```python
from build123d import *

# Parameters (mm, degrees)
SKETCH1_W           = 101.6
SKETCH1_H           = 19.05
BOSS_EXTRUDE1_DEPTH = 3.175
SKETCH2_W           = 19.05
SKETCH2_H           = 19.05
BOSS_EXTRUDE2_DEPTH = 266.7
SKETCH4_W           = 114.3
SKETCH4_H           = 114.3
BOSS_EXTRUDE3_DEPTH = 76.2
SKETCH5_W           = 25.4
SKETCH5_H           = 38.1
CUT_EXTRUDE2_DEPTH  = 150.368
SKETCH7_OUTSIDE_W   = 192.692
SKETCH7_OUTSIDE_H   = 192.692
SKETCH7_OUTSIDE_W_2 = 101.6
SKETCH7_OUTSIDE_H_2 = 101.6
CUT_EXTRUDE3_DEPTH  = 50.8
SKETCH8_W           = 25.4
SKETCH8_H           = 33.866666666
CUT_EXTRUDE4_DEPTH  = 140.208
SKETCH9_W           = 114.3
SKETCH9_H           = 114.3
CUT_EXTRUDE5_DEPTH  = 12.7
FILLET2_R           = 6.35
SKETCH10_R          = 6.35
CUT_EXTRUDE6_DEPTH  = 12.7
SCALE1_SCALE        = 0.06
MOVE_FACE1_BY       = 0.380000002
MOVE_FACE1_2_BY     = 0.380000002
SKETCH12_R          = 0.5
BOSS_EXTRUDE4_DEPTH = 0.3
BOSS_EXTRUDE5_DEPTH = 0.3


with BuildPart() as part:
    # Sketch1 → Boss-Extrude1 (new body)
    with BuildSketch(Plane(origin=(0, 0, 0), x_dir=(0, 0, -1), z_dir=(1, 0, 0))):
        Rectangle(SKETCH1_W, SKETCH1_H)
    extrude(amount=BOSS_EXTRUDE1_DEPTH)

    # Sketch2 → Boss-Extrude2 (add)
    with BuildSketch(Plane(origin=(3.175, 0, 0), x_dir=(0, 0, -1), z_dir=(1, 0, 0))):
        Rectangle(SKETCH2_W, SKETCH2_H)
    extrude(amount=BOSS_EXTRUDE2_DEPTH)

    # Sketch4 → Boss-Extrude3 (add)
    with BuildSketch(Plane(origin=(269.875, 0, 0), x_dir=(0, 0, -1), z_dir=(1, 0, 0))):
        Rectangle(SKETCH4_W, SKETCH4_H)
    extrude(amount=BOSS_EXTRUDE3_DEPTH)

    # Sketch5 → Cut-Extrude2 (cut)
    with BuildSketch(Plane.XZ.offset(57.15)):
        with Locations((282.575, 38.1)):
            Rectangle(SKETCH5_W, SKETCH5_H)
        with Locations((282.575, -38.1)):
            Rectangle(SKETCH5_W, SKETCH5_H)
    extrude(amount=-CUT_EXTRUDE2_DEPTH, mode=Mode.SUBTRACT)

    # Sketch7 outside → Cut-Extrude3 (cut)
    with BuildSketch(Plane.ZY.offset(-269.875)):
        Rectangle(SKETCH7_OUTSIDE_W, SKETCH7_OUTSIDE_H)
        Rectangle(SKETCH7_OUTSIDE_W_2, SKETCH7_OUTSIDE_H_2, mode=Mode.SUBTRACT)
    extrude(amount=-CUT_EXTRUDE3_DEPTH, mode=Mode.SUBTRACT)

    # Sketch8 → Cut-Extrude4 (cut)
    with BuildSketch(Plane.XY.offset(50.8)):
        with Locations((307.975, 0)):
            Rectangle(SKETCH8_W, SKETCH8_H)
    extrude(amount=-CUT_EXTRUDE4_DEPTH, mode=Mode.SUBTRACT)

    # Sketch9 → Cut-Extrude5 (cut)
    with BuildSketch(Plane(origin=(346.075, 0, 0), x_dir=(0, 0, -1), z_dir=(1, 0, 0))):
        Rectangle(SKETCH9_W, SKETCH9_H)
    extrude(amount=-CUT_EXTRUDE5_DEPTH, mode=Mode.SUBTRACT)

    # Fillet2
    fillet2_edges = [part.edges().sort_by_distance(p)[0] for p in [
        (327.025, -57.15, 57.15),
        (327.025, 57.15, 57.15),
        (327.025, -57.15, -57.15),
        (327.025, 57.15, -57.15),
    ]]
    fillet(fillet2_edges, radius=FILLET2_R)

    # Sketch10 → Cut-Extrude6 (cut)
    with BuildSketch(Plane.ZY):
        with Locations((-38.1, 0)):
            Circle(SKETCH10_R)
        with Locations((38.1, 0)):
            Circle(SKETCH10_R)
    extrude(amount=-CUT_EXTRUDE6_DEPTH, mode=Mode.SUBTRACT)


with BuildPart() as part_1:
    # Scale1: scaled about (275.471689012, 0, 0)
    add(part.part.scale(SCALE1_SCALE).moved(Location((258.943387671, 0, 0))))

    # Move Face1: a face moved outward by 0.38
    extrude(part_1.faces().sort_by_distance((259.038637671, 0, -3.048))[0], amount=MOVE_FACE1_BY, dir=(0, 0, -1))

    # Move Face1 2: a face moved outward by 0.38
    extrude(part_1.faces().sort_by_distance((259.038637671, 0, 3.048))[0], amount=MOVE_FACE1_2_BY, dir=(0, 0, 1))

    # Sketch12 → Boss-Extrude4 (add)
    with BuildSketch(Plane(origin=(278.945887671, 0, 0), x_dir=(0, 0, -1), z_dir=(1, 0, 0))):
        Circle(SKETCH12_R)
    extrude(amount=BOSS_EXTRUDE4_DEPTH)

    # Sketch13 → Boss-Extrude5 (add)
    with BuildSketch(Plane(origin=(279.245887671, 0, 0), x_dir=(0, 0, -1), z_dir=(1, 0, 0))):
        with BuildLine():
            Line((0.6, 0.11), (-0.6, 0.11))
            ThreePointArc((-0.6, 0.11), (0, 0.71), (0.6, 0.11))
        make_face()
        with BuildLine():
            Line((0.6, -0.11), (-0.6, -0.11))
            ThreePointArc((-0.6, -0.11), (0, -0.71), (0.6, -0.11))
        make_face()
    extrude(amount=BOSS_EXTRUDE5_DEPTH)


solid = part_1.part
```
Build history of the part. All positions in model axes, mm. A direction names the side the tool comes from. Round coordinates to 2 decimals unless told otherwise and drop trailing zeros. Write each loop counter-clockwise with the first axis right and the second up, starting at its lowest first coordinate (ties: lowest second). Pieces come first, ordered by that corner, then holes. Notation, with made-up numbers: (42, -9) - (46, -9) arc R11 ccw to (46, 1) - close; hole circle Ø3 at (39, 1.25). An arc over 180 degrees is marked (long way). Answer as CSV lines item,"result".
Q1. Drop flat-ended pins along their axis: pin 1 (0.8 mm diameter, centred on x = 275.5, y = 1, fed in from +Z); pin 2 (0.8 mm diameter, centred on x = 276, y = -0.5, fed in from -Z); pin 3 (2 mm diameter, centred on x = 265, z = -1.5, fed in from -Y); pin 4 (1 mm diameter, centred on x = 264, y = -2.5, fed in from +Z). Give the stop position or say it passes through.
Report:
pin 1,"stops at z = 1.14"
pin 2,"stops at z = -1.14"
pin 3,"stops at y = -0.57"
pin 4,"passes through"
Q2. Cut at B-B (z = 0). Write the cut outline in (x, y).
Report:
outline,"(258.94, -0.57) - (275.14, -0.57) - (275.14, -3.05) - (278.18, -3.05) - (278.18, -3.43) - (278.95, -3.43) - (278.95, -0.5) - (279.25, -0.5) - (279.25, -0.71) - (279.55, -0.71) - (279.55, -0.11) - (279.25, -0.11) - (279.25, 0.11) - (279.55, 0.11) - (279.55, 0.71) - (279.25, 0.71) - (279.25, 0.5) - (278.95, 0.5) - (278.95, 3.43) - (278.18, 3.43) - (278.18, 3.05) - (275.14, 3.05) - (275.14, 0.57) - (258.94, 0.57) - close; hole (276.66, -1.02) - (278.18, -1.02) - (278.18, 1.02) - (276.66, 1.02) - close"
Q3. Pull direction X, two halves, no side cores. Call faces 4 (the flat face through (276.66, 2, -2)), 5 (the flat face through (259.134, 0, 1.7)), 6 (the flat face through (277, -2, 3.048)): +X half, -X half, draft (parallel to the pull), parting line (faces both ways), or undercut.
Report:
face 4,"-X half"
face 5,"undercut"
face 6,"draft"
Q4. Tool access for faces 1 (the flat face through (276.66, -2, 2)), 2 (the flat face through (276.66, -2, -2)), 3 (the flat face through (276.66, 0, 0)): list every direction of +Z, -Z, +X, -X, +Y, -Y with a clear straight run to the whole face (end or side of a thin tool).
Report:
face 1,"+Z, -X, +Y, -Y"
face 2,"-Z, -X, +Y, -Y"
face 3,"+Z, -Z"
Q5. Drill centre lines: probe 1 along X at (y, z) = (-0.25, 0.25); probe 2 along X at (y, z) = (3, 1); probe 3 along X at (y, z) = (2.75, -2.75). Where is each one in solid material? Low to high. Write a range as [from, to].
Report:
probe 1,"x = [258.94, 276.66], [278.18, 279.55]"
probe 2,"x = [275.14, 278.95]"
probe 3,"x = [276.66, 278.95]"
Q6. Cut at D-D (x = 264.5). Write the cut outline in (y, z).
Report:
outline,"(-0.57, -0.57) - (0.57, -0.57) - (0.57, 0.57) - (-0.57, 0.57) - close"
Q7. Cut at C-C (y = -1.75). Write the cut outline in (x, z), and give its area (3 significant figures).
Report:
outline,"(275.14, -1.14) - (276.66, -1.14) - (276.66, -3.05) - (278.18, -3.05) - (278.18, -3.43) - (278.95, -3.43) - (278.95, 3.43) - (278.18, 3.43) - (278.18, 3.05) - (276.66, 3.05) - (276.66, 1.14) - (275.14, 1.14) - close"
area,"18.0 mm^2"
Q8. Cut at A-A (z = -1.5). Write the cut outline in (x, y), and give its area (3 significant figures).
Report:
outline,"(258.94, -0.57) - (259.13, -0.57) - (259.13, 0.57) - (258.94, 0.57) - close; (276.66, -3.05) - (278.18, -3.05) - (278.18, -3.43) - (278.95, -3.43) - (278.95, 3.43) - (278.18, 3.43) - (278.18, 3.05) - (276.66, 3.05) - (276.66, 1.02) - (278.18, 1.02) - (278.18, -1.02) - (276.66, -1.02) - close"
area,"11.6 mm^2"
